Autodesk Inventor part; units mm, degrees
ref_plane "YZ Plane" through (0, 0, 0) normal (1, 0, 0) x (0, 1, 0)
ref_plane "XZ Plane" through (0, 0, 0) normal (0, 1, 0) x (-1, 0, 0)
ref_plane "XY Plane" through (0, 0, 0) normal (0, 0, 1) x (1, 0, 0)
sketch "Sketch1" plane through (0, 0, 0) normal (0, 0, 1) x (1, 0, 0)
  line L0 (0, 0) -> (660.4, 0)
  line L1 (660.4, 0) -> (660.4, 508)
  line L2 (660.4, 508) -> (0, 508)
  line L3 (0, 508) -> (0, 0)
  dimension "d0" = 660.4
  dimension "d1" = 508
extrude "Extrusion1" add sketch "Sketch1" along normal blind 914.4
sketch "Sketch2" plane through (660.4, 0, 0) normal (1, 0, 0) x (0, 0, -1)
  circle A0 centre (-832.0024, 64.77) radius 7.3279
  line L0 (-914.4, 0) -> (-914.4, 508)
  line L1 (0, 0) -> (-914.4, 0)
  line L2 (0, 0) -> (-914.4, 0)
  line L3 (-457.2, 0) -> (-457.2, 118.7957)
  circle A1 centre (-82.3976, 64.77) radius 7.3279
  dimension "d4" = 14.6558
  dimension "d5" = 82.3976
  dimension "d6" = 64.77
extrude "Extrusion2" add sketch "Sketch2" along normal blind 59.0804
sketch "Sketch3" plane through (0, 0, 0) normal (-1, 0, 0) x (0, 0, 1)
  line L0 (0, 508) -> (0, 0)
  line L1 (0, 0) -> (914.4, 0)
  line L2 (914.4, 508) -> (914.4, 0)
  line L3 (0, 508) -> (914.4, 508)
  circle A0 centre (832.0024, 64.77) radius 7.3279
  circle A1 centre (82.3976, 64.77) radius 7.3279
extrude "Extrusion3" add sketch "Sketch3" along normal blind 59.0804 contours A0 | A1
properties part number "Frame"
Geometry check sheet. Reference: the model listing, model coordinates, mm. Round coordinates to 2 decimals unless told otherwise and drop trailing zeros. Write each loop counter-clockwise with the first axis right and the second up, starting at its lowest first coordinate (ties: lowest second). Pieces come first, ordered by that corner, then holes. Notation, with made-up numbers: (-21, 28.25) -> (29, 28.25) arc R10 cw to (29, 43.25) -> close; hole circle Ø11 at (2, 84.25). An arc over 180 degrees is marked (long way). One line per item, written item: value. Start each with the question number.
(1) Cross-section at B-B, the plane y = 214.5. Record the cut outline in (x, z).
(2) Scan lines: line 1 (X direction, y = 231.5, z = 352.5); line 2 (Z direction, x = -25.5, y = 64.5). Record each from-to range of solid material in increasing order. Write a range as [from, to].
(3) Go/stop test with flat-tipped pins: pin 1 Ø3 at (y, z) = (189, 802) entering from -X; pin 2 Ø8 at (x, z) = (604.5, 190) entering from -Y; pin 3 Ø1 at (y, z) = (427.5, 359) entering from +X. Record where each tip stops, or that it passes through.
(4) Cross-section at A-A, the plane z = 288. Record the cut outline in (x, y).
Answer:
1. outline: (0, 0) -> (660.4, 0) -> (660.4, 914.4) -> (0, 914.4) -> close
2. line 1: [0, 660.4]
2. line 2: [75.07, 89.72], [824.68, 839.33]
3. pin 1: x = 0
3. pin 2: y = 0
3. pin 3: x = 660.4
4. outline: (0, 0) -> (660.4, 0) -> (660.4, 508) -> (0, 508) -> close
